Could you check a few things on this drawing? It's one solid part, dimensions in mm from its lowest x, y, z. Coordinates: 2 decimals unless noted, no trailing zeros. Order: outer loops, then holes, each group sorted by start corner. A loop starts at its lowest first (then second) coordinate and runs counter-clockwise, first axis right, second up. Notation, with made-up numbers: (83.25, -19) -> (127.25, -19) arc R23 cw to (127.25, -6) -> close; hole circle Ø11 at (29.5, -12.75). An arc over 180 degrees is marked (long way). Use a Markdown table: item, result. Add a question column.
1. Suppose I cut it at C-C, the plane z = 200. List the corners of the cut face in (x, y) for me, then the cut area to 3 significant figures.
2. For pin 1 Ø1.5 at (x, y) = (17.5, 148) entering from +Z; pin 2 Ø2.5 at (x, y) = (25.5, 148) entering from -Z; pin 3 Ø8 at (x, y) = (40, 57) entering from +Z, each with a flat end and sliding along its axis, tell me the tip position at first contact or that it passes through.
3. We'd pull the mould along X, two halves only. Please class the marked faces 1, 2, 3 and 4: pulls with the +X half, pulls with the -X half, needs draft (parallel to the pull), parting line crosses it, or undercut.
4. Suppose I cut it at B-B, the plane z = 485. List the corners of the cut face in (x, y) for me.
5. If I drill on line 1 along X through (y, z) = (73, 375.5); line 2 along Y through (x, z) = (25, 397), over which ranges is the centre line in solid material (lowest first)? Write a range as from..to.
6. Suppose I cut it at A-A, the plane x = 28. List the corners of the cut face in (y, z) for me.
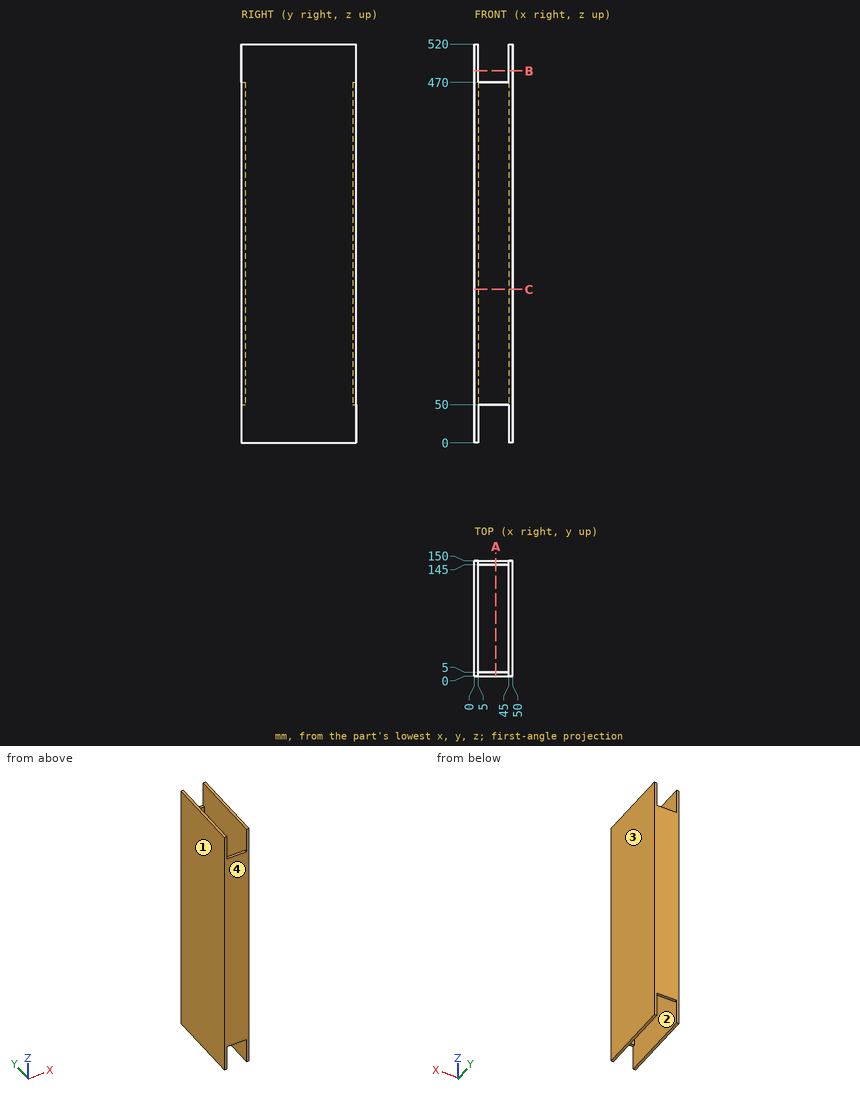
Worked out:
| question | item | result |
|---|---|---|
| 1 | outline | (0, 0) -> (50, 0) -> (50, 150) -> (0, 150) -> close; hole (5, 5) -> (45, 5) -> (45, 145) -> (5, 145) -> close |
| 1 | area | 1,900 mm² |
| 2 | pin 1 | stops at z = 470 |
| 2 | pin 2 | stops at z = 50 |
| 2 | pin 3 | passes through |
| 3 | face 1 | pulls with the -X half |
| 3 | face 2 | undercut |
| 3 | face 3 | pulls with the +X half |
| 3 | face 4 | needs draft |
| 4 | outline | (0, 0) -> (5, 0) -> (5, 150) -> (0, 150) -> close; (45, 0) -> (50, 0) -> (50, 150) -> (45, 150) -> close |
| 5 | line 1 | x = 0..5, 45..50 |
| 5 | line 2 | y = 0..5, 145..150 |
| 6 | outline | (0, 50) -> (5, 50) -> (5, 470) -> (0, 470) -> close; (145, 50) -> (150, 50) -> (150, 470) -> (145, 470) -> close |
